Geometry: final body of the model. Coordinates: model frame, mm. Face numbers are marked on the shaded views. A direction names the side the tool comes from. Give positions to 0.01 mm unless a question says otherwise; leave off trailing zeros. Write each loop counter-clockwise with the first axis right and the second up, starting at its lowest first coordinate (ties: lowest second). Pieces come first, ordered by that corner, then holes. Notation, with made-up numbers: (3, 88) -> (28, 88) arc R24 cw to (28, 126) -> close; hole circle Ø10 at (-16.5, 86.25). An arc over 180 degrees is marked (long way). Answer in a Markdown table with one row per item. Add a question column.
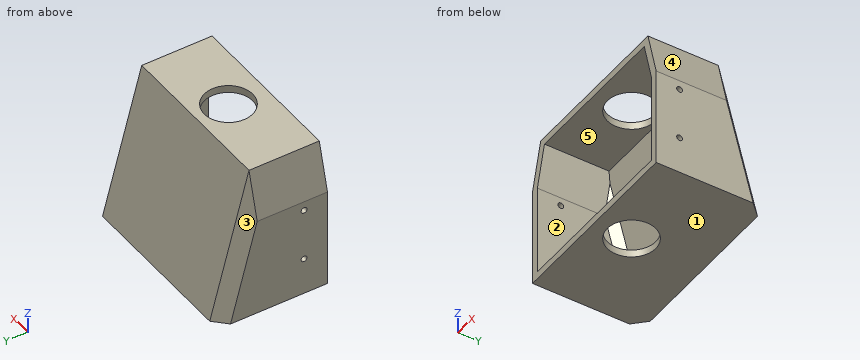
from build123d import *

# Parameters (mm, degrees)
BOSS_EXTRUDE1_DEPTH      = 60
BOSS_EXTRUDE2_DEPTH      = 70
BOSS_EXTRUDE2_DEPTH_BACK = 70
BOSS_EXTRUDE3_DEPTH      = 125
SKETCH5_W                = 177.8
SKETCH5_H                = 177.8
CUT_EXTRUDE1_DEPTH       = 206.048289966
SKETCH6_W                = 177.8
SKETCH6_H                = 177.8
CUT_EXTRUDE2_DEPTH       = 206.048289966
CUT_EXTRUDE5_START       = 93.49365
SKETCH10_W               = 39.282032303
SKETCH10_H               = 90
CUT_EXTRUDE5_DEPTH       = 247.327703168
SHELL1_T                 = -6.35
SKETCH7_R                = 20.64
CUT_EXTRUDE3_DEPTH       = 25.4
CUT_EXTRUDE4_START       = -25.4
SKETCH8_R                = 20.64
CUT_EXTRUDE4_DEPTH       = 25.4
CUT_EXTRUDE6_DEPTH       = 139.429414225
CUT_EXTRUDE6_DEPTH_BACK  = 139.429414225
SKETCH11_R               = 2.5


with BuildPart() as part:
    # Sketch1 → Boss-Extrude1 (new body)
    with BuildSketch(Plane(origin=(0, 0, 0), x_dir=(1, 0, 0), z_dir=(0, 1, 0))):
        Polygon((-103.493649054, 62.5), (103.493649054, 62.5), (70, -62.5), (-70, -62.5), align=None)
    extrude(amount=BOSS_EXTRUDE1_DEPTH)

    # Sketch2 → Boss-Extrude2 (add, two sides: drawn at the far end of the back side and taken through both)
    with BuildSketch(Plane(origin=(0, 0, 0), x_dir=(0, 0, -1), z_dir=(1, 0, 0)).offset(-BOSS_EXTRUDE2_DEPTH_BACK)):
        Polygon((-62.5, 60), (62.5, 93.493649054), (62.5, 60), align=None)
    extrude(amount=BOSS_EXTRUDE2_DEPTH + BOSS_EXTRUDE2_DEPTH_BACK)

    # Sketch4 → Boss-Extrude3 (add)
    with BuildSketch(Plane(origin=(0, 0, -62.5), x_dir=(-1, 0, 0), z_dir=(0, 0, -1))):
        Polygon((-70, 93.493649054), (-70, 60), (-103.493649054, 60), align=None)
        Polygon((70, 60), (103.493649054, 60), (70, 93.493649054), align=None)
    extrude(amount=-BOSS_EXTRUDE3_DEPTH)

    # Sketch5 → Cut-Extrude1 (cut, through all)
    with BuildSketch(Plane(origin=(70.830704378, 70.830704378, 18.979030037), x_dir=(0.7186724352001954, -0.6601192398037351, -0.21852350016499306), z_dir=(0.6947465906068516, 0.6947465906068802, 0.18615678789738468))):
        Rectangle(SKETCH5_W, SKETCH5_H)
    extrude(amount=CUT_EXTRUDE1_DEPTH, mode=Mode.SUBTRACT)

    # Sketch6 → Cut-Extrude2 (cut, through all)
    with BuildSketch(Plane(origin=(-70.830704378, 70.830704378, 18.979030037), x_dir=(0.7186724352001954, 0.6601192398037351, 0.21852350016499306), z_dir=(-0.6947465906068516, 0.6947465906068802, 0.18615678789738468))):
        Rectangle(SKETCH6_W, SKETCH6_H)
    extrude(amount=CUT_EXTRUDE2_DEPTH, mode=Mode.SUBTRACT)

    # Sketch10 → Cut-Extrude5 (cut, through all)
    with BuildSketch(Plane(origin=(0, 0, 0), x_dir=(1, 0, 0), z_dir=(0, 1, 0)).offset(CUT_EXTRUDE5_START)):
        with Locations((-100.358983849, 22.5)):
            Rectangle(SKETCH10_W, SKETCH10_H)
        with Locations((100.358983849, 22.5)):
            Rectangle(SKETCH10_W, SKETCH10_H)
    extrude(amount=-CUT_EXTRUDE5_DEPTH, mode=Mode.SUBTRACT)

    # Shell1
    shell1_openings = [part.faces().sort_by_distance(p)[0] for p in [
        (0, 0, -1.067232638),
    ]]
    offset(amount=SHELL1_T, openings=shell1_openings, kind=Kind.INTERSECTION)

    # Sketch7 → Cut-Extrude3 (cut)
    with BuildSketch(Plane(origin=(0, 0, -62.5), x_dir=(-1, 0, 0), z_dir=(0, 0, -1))):
        with Locations((0, 31.75)):
            Circle(SKETCH7_R)
    extrude(amount=-CUT_EXTRUDE3_DEPTH, mode=Mode.SUBTRACT)

    # Sketch8 → Cut-Extrude4 (cut)
    with BuildSketch(Plane.XY.offset(62.5).offset(CUT_EXTRUDE4_START)):
        with Locations(Location((0, 31.75, 0), (0, 0, 180))):
            Circle(SKETCH8_R)
    extrude(amount=CUT_EXTRUDE4_DEPTH, mode=Mode.SUBTRACT)

    # Sketch11 → Cut-Extrude6 (cut, two sides: drawn at the far end of the back side and taken through both)
    with BuildSketch(Plane(origin=(0, 0, 0), x_dir=(0, 0, -1), z_dir=(1, 0, 0)).offset(-CUT_EXTRUDE6_DEPTH_BACK)):
        with Locations((-14.5, 20)):
            Circle(SKETCH11_R)
        with Locations((30.5, 20)):
            Circle(SKETCH11_R)
    extrude(amount=CUT_EXTRUDE6_DEPTH + CUT_EXTRUDE6_DEPTH_BACK, mode=Mode.SUBTRACT)


solid = part.part
Q1. Line query: probe 1 along Z at (x, y) = (-33, 9); probe 2 along X at (y, z) = (22.5, 9); probe 3 along X at (y, z) = (12, 51.5). Output: solid intervals per line, ascending. Write a range as from..to.
Q2. Section B-B on y = 26. Return loops of the section in (x, z).
Q3. Pull-direction query (X, two-part tool) for the marked faces 1, 2 and 3; classes: +X half, -X half, draft (parallel to the pull), parting line (faces both ways), or undercut.
Q4. Section C-C on z = -30. Return loops of the section in (x, y).
Q5. Section D-D on y = 63.5. Return loops of the section in (x, z).
Q6. Contact query for flat-ended pins moving along their axis: pin 1 Ø6.5 at (y, z) = (20, 14.5) entering from +X; pin 2 Ø5 at (x, z) = (44.5, 35) entering from +Y; pin 3 Ø4 at (y, z) = (20, -30.5) entering from +X; pin 4 Ø2 at (y, z) = (42, 48.5) entering from -X. Output: stop coordinate, or through.
Q7. Section A-A on x = 0. Return loops of the section in (y, z), and give its area (3 significant figures).
Q8. Access query for the marked faces 4 and 5. Directions: +Z, -Z, +X, -X, +Y, -Y. A direction counts if a zero-diameter tool reaches every point of the face in a straight line with its end or side. Return the directions, or none.
Checks:
| question | item | result |
|---|---|---|
| 1 | probe 1 | -62.5..-56.15, 56.15..62.5 |
| 1 | probe 2 | -80.72..-74.37, 74.37..80.72 |
| 1 | probe 3 | -72.95..-66.37, 66.37..72.95 |
| 2 | outline | (-80.72, -62.5) -> (-19.82, -62.5) -> (-19.82, -56.15) -> (-74.37, -56.15) -> (-74.37, 21.66) -> (-65.13, 56.15) -> (-19.82, 56.15) -> (-19.82, 62.5) -> (-70, 62.5) -> (-80.72, 22.5) -> close; (19.82, -62.5) -> (80.72, -62.5) -> (80.72, 22.5) -> (70, 62.5) -> (19.82, 62.5) -> (19.82, 56.15) -> (65.13, 56.15) -> (74.37, 21.66) -> (74.37, -56.15) -> (19.82, -56.15) -> close |
| 3 | face 1 | draft |
| 3 | face 2 | undercut |
| 3 | face 3 | -X half |
| 4 | outline | (-80.72, 0) -> (-74.37, 0) -> (-74.37, 17.55) -> (-80.72, 17.55) -> close; (-80.72, 22.45) -> (-74.37, 22.45) -> (-74.37, 71.28) -> (-67.43, 78.21) -> (67.43, 78.21) -> (74.37, 71.28) -> (74.37, 22.45) -> (80.72, 22.45) -> (80.72, 74.07) -> (70, 84.79) -> (-70, 84.79) -> (-80.72, 74.07) -> close; (74.37, 0) -> (80.72, 0) -> (80.72, 17.55) -> (74.37, 17.55) -> close |
| 5 | outline | (-80.72, -62.5) -> (80.72, -62.5) -> (80.72, 9.44) -> (70, 49.44) -> (-70, 49.44) -> (-80.72, 9.44) -> close; hole (-74.37, -56.15) -> (74.37, -56.15) -> (74.37, -0.97) -> (67.43, 24.9) -> (-67.43, 24.9) -> (-74.37, -0.97) -> close |
| 6 | pin 1 | x = 80.72 |
| 6 | pin 2 | y = 68.04 |
| 6 | pin 3 | through |
| 6 | pin 4 | x = -74.02 |
| 7 | outline | (0, -62.5) -> (11.11, -62.5) -> (11.11, -56.15) -> (0, -56.15) -> close; (0, 56.15) -> (11.11, 56.15) -> (11.11, 62.5) -> (0, 62.5) -> close; (52.39, -62.5) -> (93.49, -62.5) -> (60, 62.5) -> (52.39, 62.5) -> (52.39, 56.15) -> (55.13, 56.15) -> (85.22, -56.15) -> (52.39, -56.15) -> close |
| 7 | area | 1,190 mm^2 |
| 8 | face 4 | +Z, +X, +Y, -Y |
| 8 | face 5 | -Y |
